Autodesk Inventor part; units mm, degrees
ref_plane "YZ Plane" through (0, 0, 0) normal (1, 0, 0) x (0, 1, 0)
ref_plane "XZ Plane" through (0, 0, 0) normal (0, 1, 0) x (-1, 0, 0)
ref_plane "XY Plane" through (0, 0, 0) normal (0, 0, 1) x (1, 0, 0)
sketch "Sketch1" plane through (0, 0, 0) normal (1, 0, 0) x (0, 1, 0)
  line L0 (7.7173, 6.935) -> (2.7173, 6.935)
  line L1 (2.7173, 6.935) -> (2.7173, 1.935)
  line L2 (2.7173, 1.935) -> (7.7173, 1.935)
  line L3 (7.7173, 1.935) -> (7.7173, 6.935)
  point P0 (0, 0)
  dimension "d0" = 5
  dimension "d1" = 5
extrude "Extrusion1" add sketch "Sketch1" along normal blind 1
sketch "Sketch2" plane through (1, 0, 0) normal (1, 0, 0) x (0, 0, -1)
  line L0 (-5.835, 6.6173) -> (-3.035, 6.6173)
  line L1 (-3.035, 6.6173) -> (-3.035, 3.8173)
  line L2 (-3.035, 3.8173) -> (-5.835, 3.8173)
  line L3 (-5.835, 3.8173) -> (-5.835, 6.6173)
  line L4 (-1.935, 7.7173) -> (-6.935, 7.7173)
  line L5 (-6.935, 7.7173) -> (-6.935, 2.7173)
  point P0 (0, 0)
  point P1 (-5.835, 5.2173)
  point P2 (-6.935, 5.2173)
  dimension "d4" = 2.8
  dimension "d5" = 2.8
  dimension "d6" = 1.1
  dimension "d7" = 1.1
extrude "Extrusion2" add sketch "Sketch2" along normal blind 11.5
fillet "Fillet1" radius 0.5 4 edges at (12.5, 5.2173, 5.835) (12.5, 6.6173, 4.435) (12.5, 5.2173, 3.035) (12.5, 3.8173, 4.435)
properties part number "Enclosure_Button"
Work out the finished part from the listing and answer in its coordinate system (mm). A direction names the side the tool comes from. Round coordinates to 2 decimals unless told otherwise and drop trailing zeros. Write each loop counter-clockwise with the first axis right and the second up, starting at its lowest first coordinate (ties: lowest second). Pieces come first, ordered by that corner, then holes.
1) A tool of negligible diameter and unlimited length cuts with its end or side. For faces 1 (the flat face through (6, 6.617, 4)), 2 (the flat face through (6, 3.817, 4)), 3 (the flat face through (0, 5, 4)), 4 (the flat face through (6, 5, 3.035)), 5 (the flat face through (6, 5, 5.835)), from which of +Z, -Z, +X, -X, +Y, -Y can it reach the whole face along a straight path? Write none if from no direction.
2) A cutting plane is placed at A-A (z = 5). Give the vertices of the cut face in (x, y), plus the area to 3 significant figures.
3) Straight lines are drawn through the part: line 1 (Y direction, x = 9.5, z = 4.3); line 2 (Z direction, x = 4, y = 6.1) (3 decimals); line 3 (X direction, y = 3.7, z = 5.45). For each, find the intervals that lie inside material, in ascending order.
4) A cutting plane is placed at D-D (z = 2.75). Give the vertices of the cut face in (x, y).
5) A cutting plane is placed at C-C (x = 2.75). Give the vertices of the cut face in (y, z) (3 decimals).
6) A cutting plane is placed at B-B (y = 4.45). Give the vertices of the cut face in (x, z) (3 decimals).
7) Given pin 1 Ø1.5 at (x, z) = (10.5, 3.5) entering from -Y; pin 2 Ø1.4 at (x, y) = (9, 4.5) entering from +Z (3 decimals); pin 3 Ø2 at (x, y) = (9, 5) entering from -Z (3 decimals), each flat-ended and moving along its own axis, determine where each tip first touches the part or whether it passes through.
Completed:
1. face 1: +Z, -Z, +X, +Y
1. face 2: +Z, -Z, +X, -Y
1. face 3: +Z, -Z, -X, +Y, -Y
1. face 4: -Z, +X, +Y, -Y
1. face 5: +Z, +X, +Y, -Y
2. outline: (0, 2.72) - (1, 2.72) - (1, 3.82) - (12, 3.82) arc R0.5 ccw to (12.5, 4.32) - (12.5, 6.12) arc R0.5 ccw to (12, 6.62) - (1, 6.62) - (1, 7.72) - (0, 7.72) - close
2. area: 37.1 mm2
3. line 1: y = 3.82 to 6.62
3. line 2: z = 3.035 to 5.835
3. line 3: x = 0 to 1
4. outline: (0, 2.72) - (1, 2.72) - (1, 7.72) - (0, 7.72) - close
5. outline: (3.817, 3.035) - (6.617, 3.035) - (6.617, 5.835) - (3.817, 5.835) - close
6. outline: (0, 1.935) - (1, 1.935) - (1, 3.035) - (12, 3.035) arc R0.5 ccw to (12.5, 3.535) - (12.5, 5.335) arc R0.5 ccw to (12, 5.835) - (1, 5.835) - (1, 6.935) - (0, 6.935) - close
7. pin 1: stops at y = 3.82
7. pin 2: stops at z = 5.835
7. pin 3: stops at z = 3.035
